Verification items for the finished model (mm, model axes). A direction names the side the tool comes from. Round coordinates to 2 decimals unless told otherwise and drop trailing zeros. Order: outer loops, then holes, each group sorted by start corner. A loop starts at its lowest first (then second) coordinate and runs counter-clockwise, first axis right, second up. Notation, with made-up numbers: (29.25, 25.5) -> (85.25, 25.5) arc R21 cw to (85.25, 62.5) -> close; hole circle Ø1 at (-32.75, 21.5). An arc over 180 degrees is marked (long way). Put each result on its own line as item: value.
```python
from build123d import *

# Parameters (mm, degrees)
EXTRUDE_769_DEPTH      = 15
SKETCH_2_R             = 9.65
CUT_EXTRUDE_1101_DEPTH = 6.15
SKETCH_3_R             = 8.65
CUT_EXTRUDE_1243_DEPTH = 33.124148841
SKETCH_4_R             = 1.35
CUT_EXTRUDE_1735_DEPTH = 11


with BuildPart() as part:
    # Эскиз1 → Extrude 769 (new, symmetric)
    with BuildSketch(Plane.XY):
        with BuildLine():
            Line((-11.912812099, 9.699737517), (-5.131711981, 12.486614118))
            ThreePointArc((-5.131711981, 12.486614118), (0, 13.5), (5.131711981, 12.486614118))
            Line((5.131711981, 12.486614118), (11.912812099, 9.699737517))
            ThreePointArc((11.912812099, 9.699737517), (13.856406461, 8), (14.356625149, 5.46692915))
            Line((14.356625149, 5.46692915), (13.379581024, -1.799114118))
            ThreePointArc((13.379581024, -1.799114118), (11.691342951, -6.75), (8.247869043, -10.6875))
            Line((8.247869043, -10.6875), (2.44381305, -15.166666667))
            ThreePointArc((2.44381305, -15.166666667), (0, -16), (-2.44381305, -15.166666667))
            Line((-2.44381305, -15.166666667), (-8.247869043, -10.6875))
            ThreePointArc((-8.247869043, -10.6875), (-11.691342951, -6.75), (-13.379581024, -1.799114118))
            Line((-13.379581024, -1.799114118), (-14.356625149, 5.46692915))
            ThreePointArc((-14.356625149, 5.46692915), (-13.856406461, 8), (-11.912812099, 9.699737517))
        make_face()
    extrude(amount=EXTRUDE_769_DEPTH, both=True)

    # Эскиз2 → Cut-Extrude 1101 (cut)
    with BuildSketch(Plane.XY.offset(15)):
        Circle(SKETCH_2_R)
    cut_extrude_1101 = extrude(amount=-CUT_EXTRUDE_1101_DEPTH, mode=Mode.SUBTRACT)

    # Mirror 1143: Cut-Extrude 1101 across plane
    add(cut_extrude_1101.mirror(Plane.XY), mode=Mode.SUBTRACT)

    # Эскиз3 → Cut-Extrude 1243 (cut, through all)
    with BuildSketch(Plane.XY.offset(8.85)):
        Circle(SKETCH_3_R)
    extrude(amount=-CUT_EXTRUDE_1243_DEPTH, mode=Mode.SUBTRACT)

    # Эскиз4 → Cut-Extrude 1735 (cut)
    with BuildSketch(Plane.XY.offset(15)):
        with Locations((-10.825317547, 6.25)):
            Circle(SKETCH_4_R)
        with Locations((0, -12.5)):
            Circle(SKETCH_4_R)
        with Locations((10.825317547, 6.25)):
            Circle(SKETCH_4_R)
    cut_extrude_1735 = extrude(amount=-CUT_EXTRUDE_1735_DEPTH, mode=Mode.SUBTRACT)

    # Mirror 1779: Cut-Extrude 1735 across plane
    add(cut_extrude_1735.mirror(Plane.XY), mode=Mode.SUBTRACT)


solid = part.part
```
Item 1: Sectioned sample at D-D, the plane y = 3.75. Record the boundary of the cut face in (x, z).
Geometry check:
outline: (-14.13, -15) -> (-8.89, -15) -> (-8.89, -8.85) -> (-7.79, -8.85) -> (-7.79, 8.85) -> (-8.89, 8.85) -> (-8.89, 15) -> (-14.13, 15) -> close; (7.79, -8.85) -> (8.89, -8.85) -> (8.89, -15) -> (14.13, -15) -> (14.13, 15) -> (8.89, 15) -> (8.89, 8.85) -> (7.79, 8.85) -> close
Item 2: Release check for a two-part mould opening along X. For faces 4 (the face through (-5.305, -12.958, 0.21)), 5 (the face through (9.204, 2.899, 11.968)), 6 (the face through (-6, -8, 15)) record: pulls with the +X half, pulls with the -X half, needs draft (parallel to the pull), parting line crosses it, or undercut.
Geometry check:
face 4: pulls with the -X half
face 5: undercut
face 6: needs draft
Item 3: Material ranges on line 1 along Y through (x, z) = (0, -10.75); line 2 along Y through (x, z) = (1, 11); line 3 along Y through (x, z) = (3.75, 12.25), recorded low to high.
Geometry check:
line 1: -16 to -13.85, -11.15 to -9.65, 9.65 to 13.5
line 2: -15.87 to -13.41, -11.59 to -9.6, 9.6 to 13.46
line 3: -14.16 to -8.89, 8.89 to 12.97
Item 4: Tool access check on faces 1 (the face through (9.204, 2.899, -11.968)), 2 (the face through (-8.57, 11.074, 0.21)), 3 (the face through (0, -12, 4)). Record the directions out of +Z, -Z, +X, -X, +Y, -Y that give a thin tool (end or side, any length) a straight path to the whole face; none if there is none.
Geometry check:
face 1: -Z
face 2: +Z, -Z, -X, +Y
face 3: +Z
Item 5: Sectioned sample at B-B, the plane x = 0. Record the boundary of the cut face in (y, z), then the cut area to 3 significant figures.
Geometry check:
outline: (-16, -15) -> (-13.85, -15) -> (-13.85, -4) -> (-11.15, -4) -> (-11.15, -15) -> (-9.65, -15) -> (-9.65, -8.85) -> (-8.65, -8.85) -> (-8.65, 8.85) -> (-9.65, 8.85) -> (-9.65, 15) -> (-11.15, 15) -> (-11.15, 4) -> (-13.85, 4) -> (-13.85, 15) -> (-16, 15) -> close; (8.65, -8.85) -> (9.65, -8.85) -> (9.65, -15) -> (13.5, -15) -> (13.5, 15) -> (9.65, 15) -> (9.65, 8.85) -> (8.65, 8.85) -> close
area: 282 mm2
Item 6: Depth check by flat-ended pin: pin 1 Ø1.6 at (x, y) = (-10.83, 6.25) entering from -Z; pin 2 Ø1.3 at (x, y) = (-11, 6) entering from +Z; pin 3 Ø2 at (x, z) = (5, 0.5) entering from +Y; pin 4 Ø15.5 at (x, y) = (3, -2) entering from +Z. Enter the tip coordinate at first touch or a pass-through.
Geometry check:
pin 1: z = -4
pin 2: z = 4
pin 3: y = 12.89
pin 4: z = 15
Item 7: Sectioned sample at A-A, the plane z = 9.5. Record the boundary of the cut face in (x, y), then the cut area to 3 significant figures.
Geometry check:
outline: (-14.36, 5.47) -> (-13.38, -1.8) arc R13.5 ccw to (-8.25, -10.69) -> (-2.44, -15.17) arc R4 ccw to (2.44, -15.17) -> (8.25, -10.69) arc R13.5 ccw to (13.38, -1.8) -> (14.36, 5.47) arc R4 ccw to (11.91, 9.7) -> (5.13, 12.49) arc R13.5 ccw to (-5.13, 12.49) -> (-11.91, 9.7) arc R4 ccw to start; hole circle Ø2.7 at (-10.83, 6.25); hole circle Ø19.3 at (0, 0); hole circle Ø2.7 at (0, -12.5); hole circle Ø2.7 at (10.83, 6.25)
area: 320 mm2
